Check sheet for the modelled part. Datum: model origin and axes. Units: mm. Give positions to 0.01 mm unless a question says otherwise; leave off trailing zeros. Order: outer loops, then holes, each group sorted by start corner. A loop starts at its lowest first (then second) coordinate and runs counter-clockwise, first axis right, second up.
Autodesk Inventor part; units mm, degrees
ref_plane "YZ Plane" through (0, 0, 0) normal (1, 0, 0) x (0, 1, 0)
ref_plane "XZ Plane" through (0, 0, 0) normal (0, 1, 0) x (-1, 0, 0)
ref_plane "XY Plane" through (0, 0, 0) normal (0, 0, 1) x (1, 0, 0)
sketch "Náčrt1" plane through (0, 0, 0) normal (0, 0, 1) x (1, 0, 0)
  point P0 (0, 0)
sketch "Náčrt2" plane through (0, 0, 0) normal (0, 0, 1) x (1, 0, 0)
  line L0 (130.81, 47.627) -> (168.91, 47.625)
  line L1 (168.91, 47.625) -> (168.91, 33.655)
  line L2 (168.91, 33.655) -> (130.81, 33.655)
  line L3 (130.81, 33.655) -> (130.81, 47.627)
  line L4 (3.81, 47.625) -> (41.91, 47.625)
  line L5 (41.91, 47.625) -> (41.91, 33.655)
  line L6 (41.91, 33.655) -> (3.81, 33.655)
  line L7 (3.81, 33.655) -> (3.81, 47.625)
  line L8 (43.18, 47.625) -> (81.28, 47.625)
  line L9 (81.28, 47.625) -> (81.28, 33.655)
  line L10 (81.28, 33.655) -> (43.18, 33.655)
  line L11 (43.18, 33.655) -> (43.18, 47.625)
  line L12 (91.44, 47.625) -> (129.54, 47.625)
  line L13 (129.54, 47.625) -> (129.54, 33.655)
  line L14 (129.54, 33.655) -> (91.44, 33.655)
  line L15 (91.44, 33.655) -> (91.44, 47.625)
  circle A0 centre (26.67, 6.35) radius 2.54
  circle A1 centre (13.97, 6.35) radius 3.81
  circle A2 centre (62.865, 11.43) radius 10.795
  circle A3 centre (114.3, 6.35) radius 2.54
  circle A4 centre (101.6, 6.35) radius 3.81
  circle A5 centre (150.495, 11.43) radius 10.795
  line L16 (31.75, 23.1775) -> (41.91, 23.1775)
  line L17 (41.91, 23.1775) -> (41.91, 17.4625)
  line L18 (41.91, 17.4625) -> (31.75, 17.4625)
  line L19 (31.75, 17.4625) -> (31.75, 23.1775)
  line L20 (119.38, 23.1775) -> (129.54, 23.1775)
  line L21 (129.54, 23.1775) -> (129.54, 17.4625)
  line L22 (129.54, 17.4625) -> (119.38, 17.4625)
  line L23 (119.38, 17.4625) -> (119.38, 23.1775)
  line L24 (0, 50.8) -> (172.72, 50.8)
  line L25 (172.72, 50.8) -> (172.72, 0)
  line L26 (172.72, 0) -> (0, 0)
  line L27 (0, 0) -> (0, 50.8)
extrude "Vysunutí1" add sketch "Náčrt2" along normal blind 2.54
properties part number "NavCom_mask"
(1) Sectioned sample at D-D (x = 48.5). Enter the section's corners in (y, z) (3 decimals).
(2) Sectioned sample at C-C (y = 38.5). Enter the section's corners in (x, z).
(3) Thickness scan on L1, parallel to Y at x = 114.3, z = 2 (3 decimals); L2, parallel to X at y = 43, z = 1.15; L3, parallel to Y at x = 94, z = 0.55 (3 decimals). Record the ranges inside material, lowest first.
(4) Release check for a two-part mould opening along Y. For faces 1 (the face through (85, 26, 2.54)), 2 (the face through (54.91, 4.13, 1.25)) record: released by +Y, released by -Y, zero draft, split by the parting line, or undercut.
(5) Sectioned sample at A-A (z = 1.1). Count the separate pieces of the cut face and the enclosed holes in it, plus the area to 3 significant figures.
(6) Sectioned sample at B-B (x = 101.6). Enter the section's corners in (y, z) (3 decimals), plus the area to 3 significant figures.
Values follow:
1. outline: (0, 0) - (33.655, 0) - (33.655, 2.54) - (0, 2.54) - close; (47.625, 0) - (50.8, 0) - (50.8, 2.54) - (47.625, 2.54) - close
2. outline: (0, 0) - (3.81, 0) - (3.81, 2.54) - (0, 2.54) - close; (41.91, 0) - (43.18, 0) - (43.18, 2.54) - (41.91, 2.54) - close; (81.28, 0) - (91.44, 0) - (91.44, 2.54) - (81.28, 2.54) - close; (129.54, 0) - (130.81, 0) - (130.81, 2.54) - (129.54, 2.54) - close; (168.91, 0) - (172.72, 0) - (172.72, 2.54) - (168.91, 2.54) - close
3. L1: y = 0 to 3.81, 8.89 to 33.655, 47.625 to 50.8
3. L2: x = 0 to 3.81, 41.91 to 43.18, 81.28 to 91.44, 129.54 to 130.81, 168.91 to 172.72
3. L3: y = 0 to 33.655, 47.625 to 50.8
4. face 1: zero draft
4. face 2: undercut
5. separate pieces: 1
5. enclosed holes: 12
5. area: 5,670 mm2
6. outline: (0, 0) - (2.54, 0) - (2.54, 2.54) - (0, 2.54) - close; (10.16, 0) - (33.655, 0) - (33.655, 2.54) - (10.16, 2.54) - close; (47.625, 0) - (50.8, 0) - (50.8, 2.54) - (47.625, 2.54) - close
6. area: 74.2 mm2
